Study the drawing (mm; zero at the part's minimum x, y, z) and answer. Round coordinates to 2 decimals unless told otherwise and drop trailing zeros. Loops run counter-clockwise (first coordinate to the right, second up) from the corner with the lowest first, then second, coordinate; pieces in that order, holes last. Notation, with made-up numbers: (71, 37) - (79, 37) arc R9 cw to (79, 51) - close; hole circle Ø2 at (46, 13). An arc over 180 degrees is marked (long way). Use CSV: the item, a comma, the result in double quotes. Start each with the question number.
1. Find section D-D (y = 13). Give the vertices of the cut face in (x, z), and give its area (3 significant figures).
2. Given pin 1 Ø2 at (x, y) = (21.5, 13) entering from -Z; pin 2 Ø8 at (x, y) = (6, 4.5) entering from +Z; pin 3 Ø5.5 at (x, y) = (14.5, 10.5) entering from -Z; pin 4 Ø0.8 at (y, z) = (9.5, 3.5) entering from +X, each flat-ended and moving along its own axis, determine where each tip first touches the part or whether it passes through.
3. Find section C-C (x = 23.5). Give the vertices of the cut face in (y, z), and give its area (3 significant figures).
4. Consider line 1 along X through (y, z) = (9.5, 0.5); line 2 along Z through (x, y) = (3.75, 9.5) (3 decimals); line 3 along Z through (x, y) = (6.5, 16). Determine where each line is inside the solid, lowest interval first.
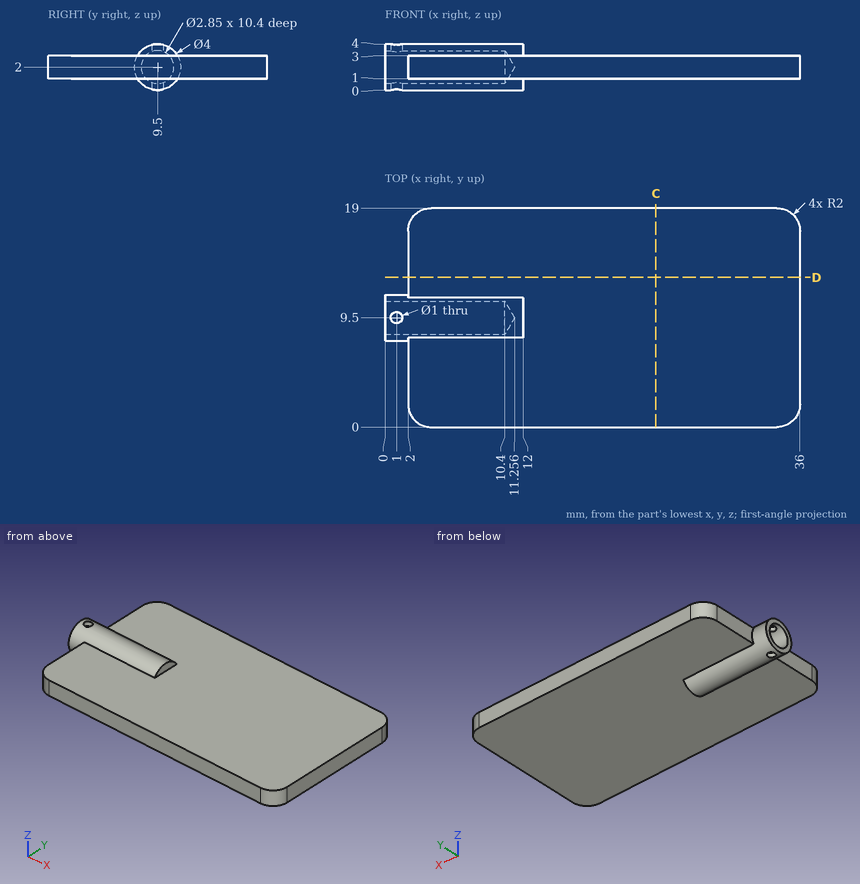
Filled sheet:
1,outline,"(2, 1) - (36, 1) - (36, 3) - (2, 3) - close"
1,area,"68.0 mm²"
2,pin 1,"stops at z = 1"
2,pin 2,"stops at z = 3.73"
2,pin 3,"stops at z = 0"
2,pin 4,"stops at x = 12"
3,outline,"(0, 1) - (19, 1) - (19, 3) - (0, 3) - close"
3,area,"38.0 mm²"
4,line 1,"x = 0 to 0.5, 1.5 to 12"
4,line 2,"z = 0 to 0.575, 3.425 to 4"
4,line 3,"z = 1 to 3"
